Geometry: final body of the model. Coordinates: model frame, mm. A direction names the side the tool comes from. Coordinates: 2 decimals unless noted, no trailing zeros. Use one line per item in the form item = value. Start each with the question number.
Autodesk Inventor part; units mm, degrees
ref_plane "YZ Plane" through (0, 0, 0) normal (1, 0, 0) x (0, 1, 0)
ref_plane "XZ Plane" through (0, 0, 0) normal (0, 1, 0) x (-1, 0, 0)
ref_plane "XY Plane" through (0, 0, 0) normal (0, 0, 1) x (1, 0, 0)
sketch "Sketch1" plane through (0, 0, 0) normal (0, 0, 1) x (1, 0, 0)
  line L0 (0, 0) -> (10, 0)
  line L1 (10, 0) -> (10, 63)
  line L2 (10, 63) -> (0, 63)
  line L3 (0, 63) -> (0, 0)
  dimension "d0" = 10
  dimension "d1" = 63
extrude "Extrusion1" add sketch "Sketch1" along normal blind 82.8
sketch "m" plane through (0, 63, 0) normal (0, 1, 0) x (1, 0, 0)
  line L0 (0, 0) -> (0, -82.8)
  line L1 (10, 0) -> (0, 0)
  point P0 (5, -41.4)
  dimension "d4" = 5
  dimension "d5" = 41.4
hole "Hole1" at (5, 63, 41.4) direction (0, -1, 0) diameter 3.242 depth 12 tip angle 118
properties part number "Paddle" material "Polypropylene"
(1) Material intervals for L1, parallel to Z at x = 5, y = 54.5; L2, parallel to X at y = 60.5, z = 41.4, sorted ascending. Write a range as from..to.
(2) Set-up query: faces 1 (the cylindrical face through (4.93, 56.92, 39.78)), 2 (the flat face through (3, 63, 41)). Return all of +Z, -Z, +X, -X, +Y, -Y with unobstructed straight access to the full face (end or side cutting, diameter ignored); none if empty.
(3) Contact query for a flat-ended pin moving along its axis: pin 1 Ø2.5 at (x, z) = (5, 41.4) entering from +Y. Output: stop coordinate, or through.
(4) Draft query along X for faces 3 (the conical face through (4.829, 50.195, 41.177)), 4 (the flat face through (10, 31, 41)), 5 (the flat face through (5, 0, 41)). Return one class per face: released by +X, released by -X, zero draft, split by the parting line, or undercut.
Check sheet entries:
q1.L1 = 0..39.78, 43.02..82.8
q1.L2 = 0..3.38, 6.62..10
q2.face_1 = +Y
q2.face_2 = +Z, -Z, +X, -X, +Y
q3.pin_1 = 50.78
q4.face_3 = undercut
q4.face_4 = released by +X
q4.face_5 = zero draft
